Study the drawing (mm; zero at the part's minimum x, y, z) and answer. Coordinates: 2 decimals unless noted, no trailing zeros. Write each loop counter-clockwise with the first axis right and the second up, starting at its lowest first coordinate (ties: lowest second). Pieces come first, ordered by that corner, then holes. Notation, with made-up numbers: (-15.75, 64) -> (-8.75, 64) arc R29 ccw to (-8.75, 99) -> close; hole circle Ø5 at (-5, 75). An arc over 180 degrees is marked (long way). Answer in a Markdown table with one row per item. Add a question column.
Item 1: Section B-B on x = 2 is taken. Count the separate pieces of the cut face and the enclosed holes in it, then the cut area to 3 significant figures.
Item 2: Section D-D on z = 20.5 is taken. Write down the section's boundary in (x, y).
Item 3: Given pin 1 Ø6 at (y, z) = (20, 19.5) entering from -X; pin 2 Ø1 at (x, z) = (2, 7) entering from +Y; pin 3 Ø1 at (x, y) = (1.5, 80) entering from -Z, each flat-ended and moving along its own axis, determine where each tip first touches the part or whether it passes through.
Item 4: Section C-C on y = 38.1 is taken. Write down the section's boundary in (x, z).
Item 5: Straight lines are drawn through the part: line 1 (Y direction, x = 1.5, z = 58.5); line 2 (Y direction, x = 2.25, z = 12.7) (1 decimal); line 3 (Z direction, x = 3.75, y = 38.1). For each, find the intervals that lie inside material, in ascending order. Write a range as from..to.
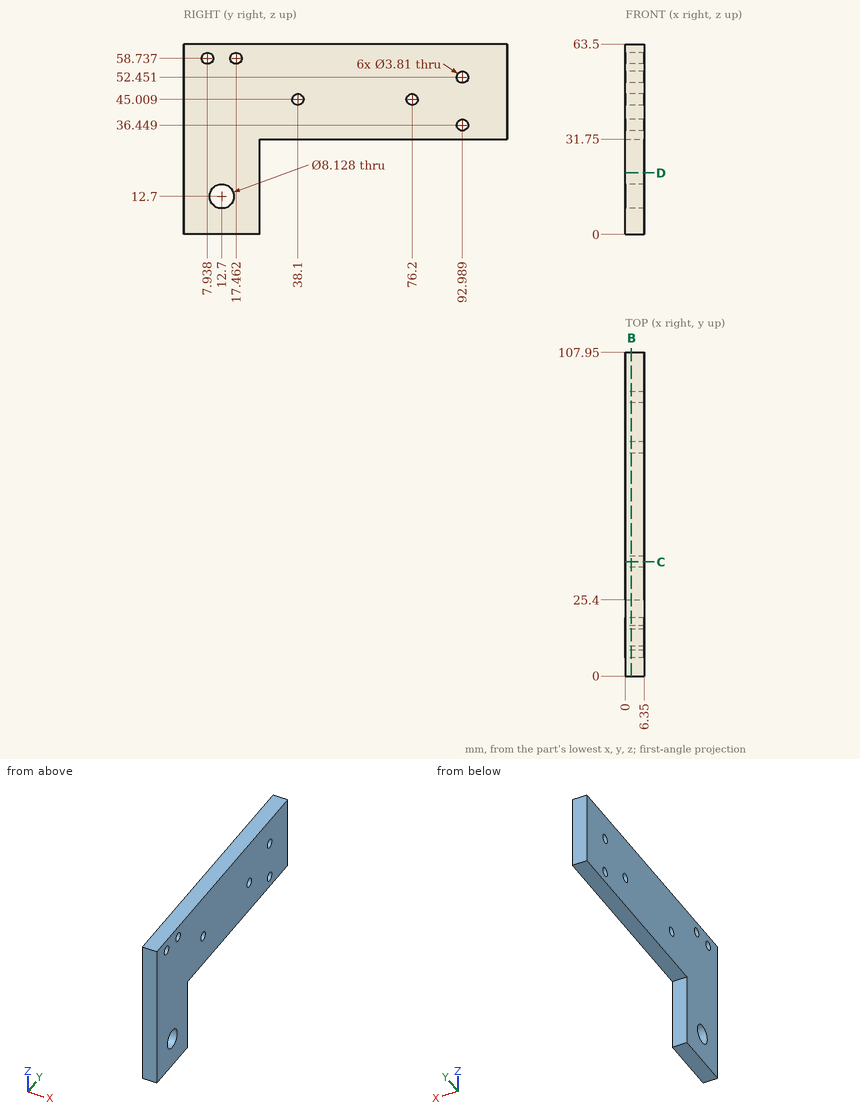
Results below:
| question | item | result |
|---|---|---|
| 1 | separate pieces | 1 |
| 1 | enclosed holes | 7 |
| 1 | area | 4,110 mm2 |
| 2 | outline | (0, 0) -> (6.35, 0) -> (6.35, 25.4) -> (0, 25.4) -> close |
| 3 | pin 1 | stops at x = 0 |
| 3 | pin 2 | stops at y = 25.4 |
| 3 | pin 3 | stops at z = 31.75 |
| 4 | outline | (0, 31.75) -> (6.35, 31.75) -> (6.35, 43.1) -> (0, 43.1) -> close; (0, 46.91) -> (6.35, 46.91) -> (6.35, 63.5) -> (0, 63.5) -> close |
| 5 | line 1 | y = 0..6.05, 9.83..15.57, 19.35..107.95 |
| 5 | line 2 | y = 0..8.6, 16.8..25.4 |
| 5 | line 3 | z = 31.75..43.1, 46.91..63.5 |
